The figure shows three views and two pictorial views of one solid part (mm, origin at its lowest corner). Answer the questions. Coordinates: 2 decimals unless noted, no trailing zeros. Write each loop counter-clockwise with the first axis right and the second up, starting at its lowest first coordinate (ties: lowest second). Pieces come first, ordered by that corner, then holes.
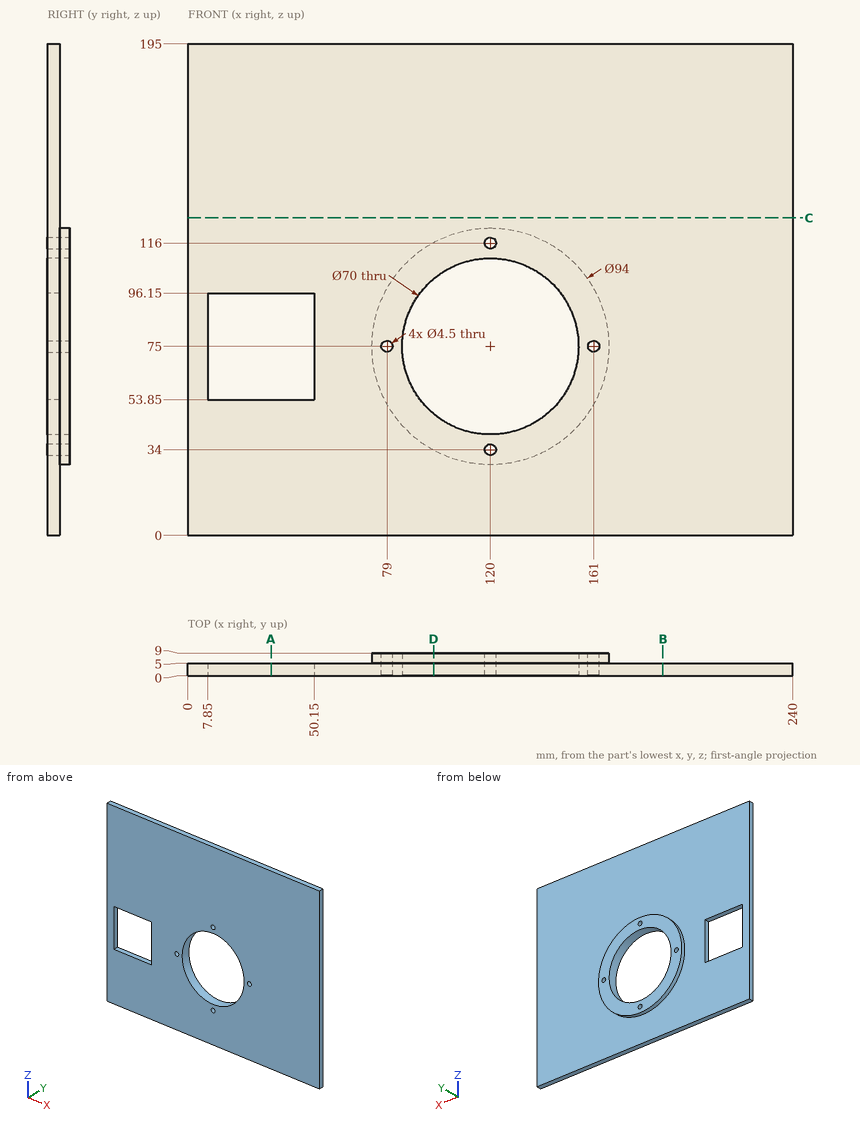
Q1. The part is cut by section A-A, the plane x = 33. Write down the section's boundary in (y, z), then the cut area to 4 significant figures.
Answers below:
outline: (0, 0) - (5, 0) - (5, 53.85) - (0, 53.85) - close; (0, 96.15) - (5, 96.15) - (5, 195) - (0, 195) - close
area: 763.5 mm2
Q2. Given pin 1 (4 mm diameter, centred on x = 120, z = 34, fed in from +Y); pin 2 (10 mm diameter, centred on x = 58.5, z = 107.5, fed in from +Y), each flat-ended and moving along its own axis, determine where each tip first touches the part or whether it passes through.
Answers below:
pin 1: passes through
pin 2: stops at y = 5
Q3. The part is cut by section D-D, the plane x = 97.5. Write down the section's boundary in (y, z), then the cut area to 3 significant figures.
Answers below:
outline: (0, 0) - (5, 0) - (5, 33.74) - (9, 33.74) - (9, 48.19) - (0, 48.19) - close; (0, 101.81) - (9, 101.81) - (9, 116.26) - (5, 116.26) - (5, 195) - (0, 195) - close
area: 823 mm2
Q4. The part is cut by section C-C, the plane z = 126. Write down the section's boundary in (x, y), then the cut area to 3 significant figures.
Answers below:
outline: (0, 0) - (240, 0) - (240, 5) - (0, 5) - close
area: 1,200 mm2
Q5. The part is cut by section B-B, the plane x = 188.5. Write down the section's boundary in (y, z), then the cut area to 3 significant figures.
Answers below:
outline: (0, 0) - (5, 0) - (5, 195) - (0, 195) - close
area: 975 mm2
Q6. Find the intervals of material crossed by probe 1 along X at (y, z) = (1.25, 74.5); probe 2 along Z at (x, y) = (121.5, 3.25); probe 3 along Z at (x, y) = (46, 3.25), in increasing order.
Answers below:
probe 1: x = 0 to 7.85, 50.15 to 76.81, 81.19 to 85, 155 to 158.81, 163.19 to 240
probe 2: z = 0 to 32.32, 35.68 to 40.03, 109.97 to 114.32, 117.68 to 195
probe 3: z = 0 to 53.85, 96.15 to 195
